from build123d import *

# Parameters (mm, degrees)
F1_DEPTH = 38.1
F2_T     = -2.54


with BuildPart() as f1:
    # F0 (on Top) → F1 (new body)
    with BuildSketch(Plane.XY):
        with BuildLine():
            ThreePointArc((-42.367201, 0), (-6.248401, -16.178203), (29.870398, 0))
            ThreePointArc((29.870398, 0), (-6.248401, 17.891403), (-42.367201, 0))
        make_face()
    extrude(amount=F1_DEPTH)

    # F2
    f2_openings = [f1.faces().sort_by_distance(p)[0] for p in [
        (-6.248401, 0.736182, 38.1),
    ]]
    offset(amount=F2_T, openings=f2_openings)


solid = f1.part
Input: part model. Units: mm. Frame: model coordinates. A direction names the side the tool comes from. Coordinates: 2 decimals unless noted, no trailing zeros. Write each loop counter-clockwise with the first axis right and the second up, starting at its lowest first coordinate (ties: lowest second). Pieces come first, ordered by that corner, then holes. Notation, with made-up numbers: M 40,47 L 52,47 A18 cw 52,64 Z; hole C 33.5,44.25 d8. An arc over 180 degrees is marked long. Answer as a JSON object with one key per item and string values. Group by question number.
(1) Section C-C on x = -35. Output: boundary loops of the cut face in (y, z).
(2) Contact query for flat-ended pins moving along their axis: P1, Ø1, axis at x = -18.5, z = 31.5, coming from the -Y side; P2, Ø8.5, axis at x = -9, y = -3.5, coming from the +Z side; P3, Ø2, axis at y = 4.5, z = 32.5, coming from the +X side. Output: stop coordinate, or through.
(3) Section B-B on z = 19.5. Output: boundary loops of the cut face in (x, y), plus the area to 3 significant figures.
(4) Ray query, line 1 along Z through (x, y) = (-15, -3.5); line 2 along X through (y, z) = (5.5, 36); line 3 along Y through (x, z) = (6, 10). Return the intervals inside material, ascending. Write a range as [from, to].
(5) Mould query, pull axis X, two halves, no side actions, for faces 1 (the face through (-7, 1, 0)), 2 (the face through (-7, 1, 2.54)), 3 (the face through (-5.73, 15.35, 20.07)), 4 (the face through (-6.819, -16.175, 18.783)). Classes: pulls with the +X half, pulls with the -X half, needs draft (parallel to the pull), parting line crosses it, or undercut.
(6) Set-up query: faces 5 (the face through (-6.759, -13.635, 20.071)), 6 (the face through (-6, -14, 38.1)). Return all of +Z, -Z, +X, -X, +Y, -Y with unobstructed straight access to the full face (end or side cutting, diameter ignored); none if empty.
(7) Section A-A on y = 10. Output: boundary loops of the cut face in (x, z), plus the area to 3 significant figures.
Result set:
{
 "1": {"outline": "M -6.71,0 L 7.63,0 L 7.63,38.1 L 4.28,38.1 L 4.28,2.54 L -3.51,2.54 L -3.51,38.1 L -6.71,38.1 Z"},
 "2": {"P1": "stops at y = -14.73", "P2": "stops at z = 2.54", "P3": "stops at x = 26.91"},
 "3": {"outline": "M -42.37,0 A48.41 ccw 29.87,0 A45.4 ccw Z; hole M -39.01,0.13 A45.87 ccw 26.51,0.13 A42.86 ccw Z", "area": "397 mm2"},
 "4": {"line 1": "z = [0, 2.54]", "line 2": "x = [-37.42, -33.59], [21.09, 24.92]", "line 3": "y = [-14.6, -11.97], [13.56, 16.21]"},
 "5": {"face 1": "needs draft", "face 2": "undercut", "face 3": "undercut", "face 4": "parting line crosses it"},
 "6": {"face 5": "+Z", "face 6": "+Z, +X, -X, +Y, -Y"},
 "7": {"outline": "M -31.83,0 L 19.33,0 L 19.33,38.1 L 14.49,38.1 L 14.49,2.54 L -26.99,2.54 L -26.99,38.1 L -31.83,38.1 Z", "area": "474 mm2"}
}
